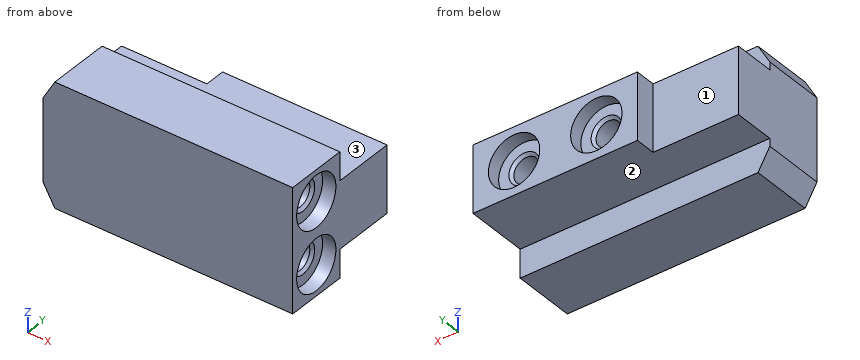
from build123d import *

# Parameters (mm, degrees)
BOSS_EXTRUDE1_DEPTH = 24.3
SKETCH2_W           = 12
SKETCH2_H           = 2
CUT_EXTRUDE1_DEPTH  = 8.3
CUT_EXTRUDE2_DEPTH  = 6


with BuildPart() as part:
    # Sketch1 → Boss-Extrude1 (new body)
    with BuildSketch(Plane(origin=(0, 0, 0), x_dir=(0, 0, -1), z_dir=(1, 0, 0))):
        Polygon((-6, 6), (-6, 0), (6, 0), (6, 6), (3.25, 6), (3.25, 12), (-3.25, 12), (-3.25, 6), align=None)
    extrude(amount=BOSS_EXTRUDE1_DEPTH)

    # Sketch2 → Cut-Extrude1 (cut)
    with BuildSketch(Plane(origin=(0, 0, 0), x_dir=(0, 0, -1), z_dir=(1, 0, 0))):
        with Locations((0, 11)):
            Rectangle(SKETCH2_W, SKETCH2_H)
    extrude(amount=CUT_EXTRUDE1_DEPTH, mode=Mode.SUBTRACT)

    # Sketch3 → Cut-Revolve1 (revolve, cut)
    with BuildSketch(Plane(origin=(0, 3, 0), x_dir=(1, 0, 0), z_dir=(0, 1, 0))):
        Polygon((15.140147844, 3), (15.85, 4.2295), (22.7295, 4.2295), (23, 4.5), (23, 5.5), (24.3, 5.5), (24.3, 3), align=None)
    revolve(axis=Axis((24.3, 3, -3), (-1, 0, 0)), mode=Mode.SUBTRACT)

    # Sketch4 → Cut-Revolve2 (revolve, cut)
    with BuildSketch(Plane(origin=(0, 3, 0), x_dir=(1, 0, 0), z_dir=(0, 1, 0))):
        Polygon((15.140147844, -3), (15.85, -1.7705), (22.7295, -1.7705), (23, -1.5), (23, -0.5), (24.3, -0.5), (24.3, -3), align=None)
    revolve(axis=Axis((24.3, 3, 3), (-1, 0, 0)), mode=Mode.SUBTRACT)

    # Sketch5 → Cut-Revolve3 (revolve, cut)
    with BuildSketch(Plane.XY):
        Polygon((20.3, 12), (22.8, 12), (22.8, 10.7), (21.8, 10.7), (21.5295, 10.4295), (21.5295, 3.55), (20.3, 2.840147844), align=None)
    revolve(axis=Axis((20.3, 2.840147844, 0), (0, 1, 0)), mode=Mode.SUBTRACT)

    # Sketch6 → Cut-Revolve4 (revolve, cut)
    with BuildSketch(Plane.XY):
        Polygon((12.3, 12), (14.8, 12), (14.8, 10.7), (13.8, 10.7), (13.5295, 10.4295), (13.5295, 3.55), (12.3, 2.840147844), align=None)
    revolve(axis=Axis((12.3, 2.840147844, 0), (0, 1, 0)), mode=Mode.SUBTRACT)

    # Sketch7 → Cut-Extrude2 (cut)
    with BuildSketch(Plane(origin=(0, 0, 0), x_dir=(1, 0, 0), z_dir=(0, 1, 0))):
        Polygon((-1, -7), (11.15, -7), (11.15, -6), (1.154700538, -6), (0, -4), (0, 4), (1.154700538, 6), (11.15, 6), (11.15, 7), (-1, 7), align=None)
    extrude(amount=CUT_EXTRUDE2_DEPTH, mode=Mode.SUBTRACT)


solid = part.part
Could you check a few things on this model? Use its own coordinates, in mm. Face numbers are marked on the shaded views. A direction names the side the tool comes from. Coordinates: 2 decimals unless noted, no trailing zeros. Order: outer loops, then holes, each group sorted by start corner. A loop starts at its lowest first (then second) coordinate and runs counter-clockwise, first axis right, second up. Notation, with made-up numbers: (40.5, 0) -> (57.5, 0) arc R11 cw to (57.5, 11) -> close; hole circle Ø8 at (-9.5, 39.5). An arc over 180 degrees is marked (long way). One line per item, written item: value. Start each with the question number.
1) Imagine slicing it at A-A on y = 9. List the corners of the cut face in (x, z) for me.
2) I'm going to push flat-ended pins straight in: pin 1 (5 mm diameter, centred on x = 6.5, y = 9, fed in from -Z); pin 2 (1.4 mm diameter, centred on x = 7, z = 4.5, fed in from +Y); pin 3 (1 mm diameter, centred on y = 9.5, z = 4.5, fed in from -X); pin 4 (0.6 mm diameter, centred on y = 11, z = 0, fed in from -X). Where does each tip first touch, or does it pass through?
3) Imagine slicing it at C-C on z = -5. List the corners of the cut face in (x, y) for me.
4) If I drill on L1, parallel to X at y = 11.6, z = 0; L2, parallel to X at y = 6, z = 0; L3, parallel to Z at x = 18, y = 3, over which ranges is the centre line in solid material (lowest first)? Write a range as [from, to].
5) Imagine slicing it at D-D on x = 21.25. Count the separate pieces of the cut face and the enclosed holes in it, plus the area to 3 significant figures.
6) Imagine slicing it at B-B on x = 8.75. List the corners of the cut face in (y, z) for me.
7) Which directions (+Z, -Z, +X, -X, +Y, -Y) give clear straight access to the entire face, cutting with the end or side of a thin tool? Please do the marked faces 1, 2 and 3.
Answer list:
1. outline: (0, -3.25) -> (24.3, -3.25) -> (24.3, 3.25) -> (0, 3.25) -> close; hole circle Ø2.46 at (12.3, 0); hole circle Ø2.46 at (20.3, 0)
2. pin 1: stops at z = -3.25
2. pin 2: stops at y = 6
2. pin 3: passes through
2. pin 4: stops at x = 8.3
3. outline: (0.58, 0) -> (24.3, 0) -> (24.3, 1.5) -> (23, 1.5) -> (23, 4.5) -> (24.3, 4.5) -> (24.3, 6) -> (0.58, 6) -> close
4. L1: x = [8.3, 9.8], [14.8, 17.8], [22.8, 24.3]
4. L2: x = [0, 11.07], [13.53, 19.07], [21.53, 24.3]
4. L3: z = [-6, -4.23], [-1.77, 1.77], [4.23, 6]
5. separate pieces: 1
5. enclosed holes: 2
5. area: 84.1 mm2
6. outline: (0, -6) -> (6, -6) -> (6, -3.25) -> (12, -3.25) -> (12, 3.25) -> (6, 3.25) -> (6, 6) -> (0, 6) -> close
7. face 1: +Z, -Z, -X, +Y
7. face 2: -Z, +X, -X, +Y
7. face 3: +Z, +X, -X, +Y
